Geometry: see drawing. Coordinates: mm, zero at the bounding-box minimum. Coordinates: 2 decimals unless noted, no trailing zeros. Loops run counter-clockwise (first coordinate to the right, second up) from the corner with the lowest first, then second, coordinate; pieces in that order, holes last. Notation, with made-up numbers: (-39.5, 40) - (12.5, 40) arc R16 cw to (12.5, 44) - close; hole circle Ø11 at (-27, 5). An arc over 180 degrees is marked (long way). Answer in a Markdown table with one row per item.
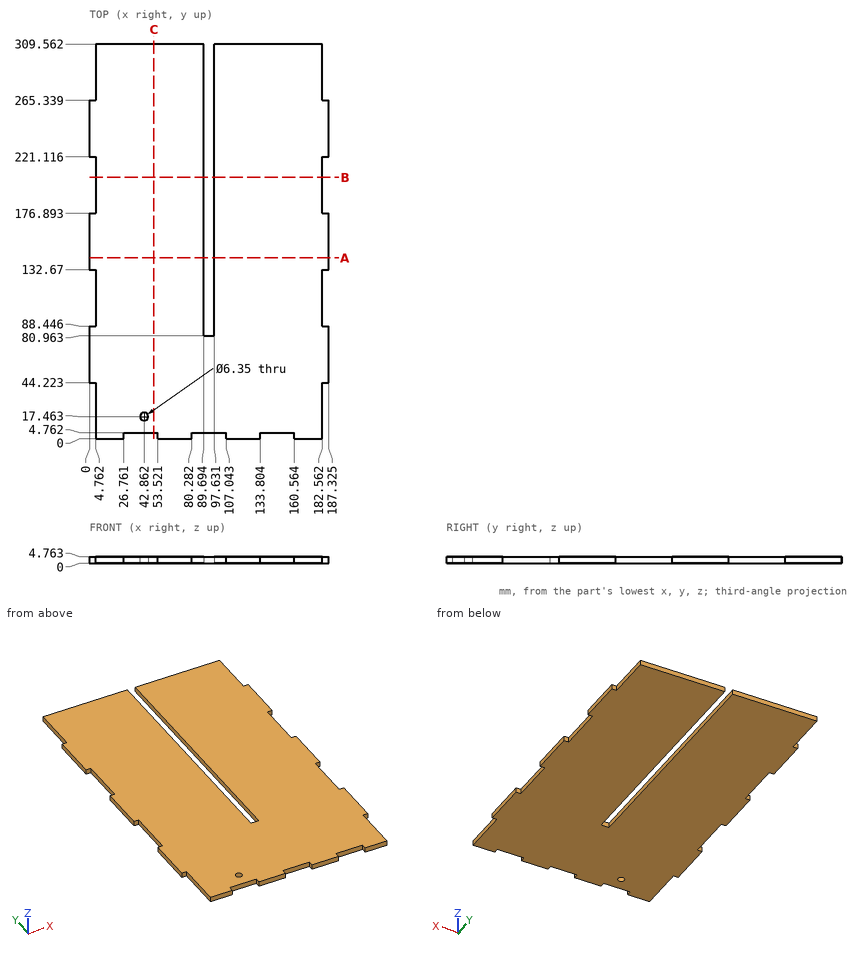
(1) Ray query, probe 1 along X at (y, z) = (205.5, 2.2); probe 2 along Y at (x, z) = (87.5, 1.8); probe 3 along X at (y, z) = (169, 1.05) (1 decimal). Return the intervals inside material, ascending.
Verdict:
| item | result |
|---|---|
| probe 1 | x = 4.76 to 89.69, 97.63 to 182.56 |
| probe 2 | y = 4.76 to 309.56 |
| probe 3 | x = 0 to 89.7, 97.6 to 187.3 |
(2) Cut plane C-C on x = 50.5. Output: boundary loops of the cut face in (y, z), then the cut area to 3 significant figures.
Verdict:
| item | result |
|---|---|
| outline | (4.76, 0) - (309.56, 0) - (309.56, 4.76) - (4.76, 4.76) - close |
| area | 1,450 mm² |
(3) First-contact query: pin 1 Ø2.5 at (x, z) = (1.5, 3) entering from -Y; pin 2 Ø1.5 at (y, z) = (64, 4) entering from -X; pin 3 Ø1.4 at (y, z) = (289, 2) entering from +X; pin 4 Ø2.5 at (x, z) = (186, 2.5) entering from +Y. Flat tips, straight axial feed; report the tip coordinate or a pass-through.
Verdict:
| item | result |
|---|---|
| pin 1 | stops at y = 44.22 |
| pin 2 | stops at x = 0 |
| pin 3 | stops at x = 182.56 |
| pin 4 | stops at y = 265.34 |
(4) Cut plane B-B on y = 205. Output: boundary loops of the cut face in (x, z), then the cut area to 3 significant figures.
Verdict:
| item | result |
|---|---|
| outline | (4.76, 0) - (89.69, 0) - (89.69, 4.76) - (4.76, 4.76) - close; (97.63, 0) - (182.56, 0) - (182.56, 4.76) - (97.63, 4.76) - close |
| area | 809 mm² |
(5) Cut plane A-A on y = 142. Output: boundary loops of the cut face in (x, z) (1 decimal).
Verdict:
| item | result |
|---|---|
| outline | (0, 0) - (89.7, 0) - (89.7, 4.8) - (0, 4.8) - close; (97.6, 0) - (187.3, 0) - (187.3, 4.8) - (97.6, 4.8) - close |
